Check sheet for the modelled part. Datum: model origin and axes. Units: mm. Face numbers are marked on the shaded views. A direction names the side the tool comes from. Round coordinates to 2 decimals unless told otherwise and drop trailing zeros. Write each loop counter-clockwise with the first axis right and the second up, starting at its lowest first coordinate (ties: lowest second). Pieces come first, ordered by that corner, then holes. Notation, with made-up numbers: (-23.5, 32) - (-13.5, 32) arc R11 ccw to (-13.5, 43) - close; hole circle Ø11 at (65.25, 20). An arc over 180 degrees is marked (long way). Use one line per item in the form item = value. Start each with the question number.
1) Section check B-B (y = -16). Record the boundary of the cut face in (x, z), then the cut area to 3 significant figures.
2) Section check C-C (x = 27). Record the boundary of the cut face in (y, z), then the cut area to 3 significant figures.
3) Section check D-D (y = 5). Record the boundary of the cut face in (x, z) (3 decimals), then the cut area to 3 significant figures.
4) Section check A-A (z = -4). Record the boundary of the cut face in (x, y), then the cut area to 3 significant figures.
5) Gauge pin test, flat ends, axial feed: P1, Ø3, axis at x = 17, z = -0.5, coming from the -Y side; P2, Ø1, axis at x = 33, z = -1, coming from the +Y side; P3, Ø11, axis at y = -14.5, z = 2.5, coming from the -X side; P4, Ø8, axis at x = 26, y = -9, coming from the +Z side. Record the tip position at first contact, or that the pin passes through.
6) Set-up check for the marked faces 1, 2, 3, 4 and 5: record each of +Z, -Z, +X, -X, +Y, -Y from which the full face is reachable in a straight line by a thin tool's end or side.
7) Scan lines: probe 1 along X at (y, z) = (3.25, 0); probe 2 along X at (y, z) = (-1, 0); probe 3 along Z at (x, y) = (17.45, 3.5). Record each from-to range of solid material in increasing order.
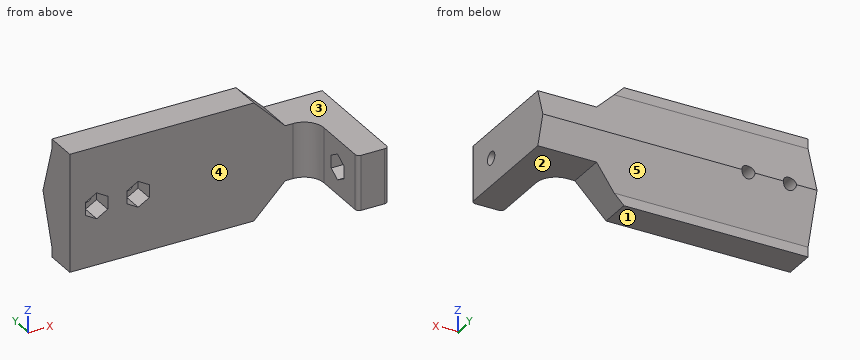
from build123d import *

# Parameters (mm, degrees)
BOSS_EXTRUDE1_DEPTH = 70
SKETCH2_R           = 1.65
CUT_EXTRUDE1_DEPTH  = 5
SKETCH3_R           = 1.65
CUT_EXTRUDE2_DEPTH  = 61
SKETCH4_W           = 8
SKETCH4_H           = 30
BOSS_EXTRUDE2_DEPTH = 20
SKETCH5_R           = 1.65
CUT_EXTRUDE3_DEPTH  = 4
SKETCH6_R           = 1.65
CUT_EXTRUDE4_DEPTH  = 40
FILLET1_R           = 1
FILLET2_R           = 5
SKETCH7_W           = 6
SKETCH7_H           = 8
SKETCH7_W_2         = 1
CUT_EXTRUDE5_DEPTH  = 42
CHAMFER1_SIZE       = 10


with BuildPart() as part:
    # Sketch1 → Boss-Extrude1 (new body)
    with BuildSketch(Plane(origin=(0, 0, 0), x_dir=(0, 0, -1), z_dir=(1, 0, 0))):
        Polygon((0, 8), (12.5, 4), (-12.5, 4), align=None)
        Polygon((12.5, 4), (-12.5, 4), (-15, 4), (-15, -4), (15, -4), (15, 4), align=None)
    extrude(amount=BOSS_EXTRUDE1_DEPTH)

    # Sketch2 → Cut-Extrude1 (cut)
    # profile 1 of 2: a face of its own
    with BuildSketch(Plane.XZ.offset(4)):
        Polygon((6.85, 3.290896534), (4, 1.645448267), (4, -1.645448267), (6.85, -3.290896534), (9.7, -1.645448267), (9.7, 1.645448267), align=None)
        with Locations(Location((6.85, 0, 0), (0, 0, 270))):
            Circle(SKETCH2_R, mode=Mode.SUBTRACT)
    # profile 2 of 2: a face of its own
    with BuildSketch(Plane.XZ.offset(4)):
        Polygon((17.45, -3.290896534), (20.3, -1.645448267), (20.3, 1.645448267), (17.45, 3.290896534), (14.6, 1.645448267), (14.6, -1.645448267), align=None)
        with Locations(Location((17.45, 0, 0), (0, 0, 270))):
            Circle(SKETCH2_R, mode=Mode.SUBTRACT)
    extrude(amount=-CUT_EXTRUDE1_DEPTH, mode=Mode.SUBTRACT)

    # Sketch3 → Cut-Extrude2 (cut)
    with BuildSketch(Plane.XZ.offset(4)):
        with Locations(Location((6.85, 0, 0), (0, 0, 270))):
            Circle(SKETCH3_R)
        with Locations(Location((17.45, 0, 0), (0, 0, 270))):
            Circle(SKETCH3_R)
    extrude(amount=-CUT_EXTRUDE2_DEPTH, mode=Mode.SUBTRACT)

    # Sketch4 → Boss-Extrude2 (add)
    with BuildSketch(Plane.XZ.offset(4)):
        with Locations((66, 0)):
            Rectangle(SKETCH4_W, SKETCH4_H)
    extrude(amount=BOSS_EXTRUDE2_DEPTH)

    # Sketch5 → Cut-Extrude3 (cut)
    with BuildSketch(Plane.ZY.offset(-62)):
        Polygon((3.290896534, -15.15), (1.645448267, -12.3), (-1.645448267, -12.3), (-3.290896534, -15.15), (-1.645448267, -18), (1.645448267, -18), align=None)
        with Locations((0, -15.15)):
            Circle(SKETCH5_R, mode=Mode.SUBTRACT)
    extrude(amount=-CUT_EXTRUDE3_DEPTH, mode=Mode.SUBTRACT)

    # Sketch6 → Cut-Extrude4 (cut)
    with BuildSketch(Plane.ZY.offset(-62)):
        with Locations((0, -15.15)):
            Circle(SKETCH6_R)
    extrude(amount=-CUT_EXTRUDE4_DEPTH, mode=Mode.SUBTRACT)

    # Fillet1
    fillet1_edges = [part.edges().sort_by_distance(p)[0] for p in [
        (70, -24, 0),
        (62, -24, 0),
    ]]
    fillet(fillet1_edges, radius=FILLET1_R)

    # Fillet2
    fillet2_edges = [part.edges().sort_by_distance(p)[0] for p in [
        (62, -4, 0),
    ]]
    fillet(fillet2_edges, radius=FILLET2_R)

    # Sketch7 → Cut-Extrude5 (cut)
    with BuildSketch(Plane.XZ.offset(24)):
        with Locations((66, 11)):
            Rectangle(SKETCH7_W, SKETCH7_H)
        with Locations((69.5, 11)):
            Rectangle(SKETCH7_W_2, SKETCH7_H)
        with Locations((60, 11)):
            Rectangle(SKETCH7_W, SKETCH7_H)
        with Locations((60, -11)):
            Rectangle(SKETCH7_W, SKETCH7_H)
        with Locations((66, -11)):
            Rectangle(SKETCH7_W, SKETCH7_H)
        with Locations((69.5, -11)):
            Rectangle(SKETCH7_W_2, SKETCH7_H)
    extrude(amount=-CUT_EXTRUDE5_DEPTH, mode=Mode.SUBTRACT)

    # Chamfer1
    # the kernel refuses this chamfer: 10 mm, written as the material it takes off along each edge
    with BuildSketch(Plane(origin=(57, -29.71682988, 15), x_dir=(0.027495876610587014, 0, -0.9996219169112968), z_dir=(0, 1, 0))) as chamfer1_piece_1_section:
        Polygon((CHAMFER1_SIZE * 0.999621916911, CHAMFER1_SIZE * 0.0274958766106), (-CHAMFER1_SIZE * 0.0274958766106, CHAMFER1_SIZE * 0.999621916911), (0, 0), align=None)
    chamfer1_piece_1 = extrude(amount=59.433659759, mode=Mode.PRIVATE)
    chamfer1_piece_1 = split(chamfer1_piece_1, bisect_by=Plane(origin=(53.542815877, 0, 7), z_dir=(0, 0, 1)), keep=Keep.TOP, mode=Mode.PRIVATE)
    add(chamfer1_piece_1, mode=Mode.SUBTRACT)
    with BuildSketch(Plane(origin=(57, -29.71682988, -15), x_dir=(-0.9996219169112968, 0, -0.027495876610586317), z_dir=(0, 1, 0))) as chamfer1_piece_2_section:
        Polygon((CHAMFER1_SIZE * 0.999621916911, CHAMFER1_SIZE * 0.0274958766106), (-CHAMFER1_SIZE * 0.0274958766106, CHAMFER1_SIZE * 0.999621916911), (0, 0), align=None)
    chamfer1_piece_2 = extrude(amount=59.433659759, mode=Mode.PRIVATE)
    chamfer1_piece_2 = split(chamfer1_piece_2, bisect_by=Plane(origin=(53.542815877, 0, -7), z_dir=(0, 0, -1)), keep=Keep.TOP, mode=Mode.PRIVATE)
    add(chamfer1_piece_2, mode=Mode.SUBTRACT)


solid = part.part
Results are:
q1.outline = (62, -7) - (70, -7) - (70, -1.41) - (66, -1.41) - (66, -2.8) - (62, -2.8) - close; (62, 2.8) - (66, 2.8) - (66, 1.41) - (70, 1.41) - (70, 7) - (62, 7) - close
q1.area = 78.3 mm²
q2.outline = (-4, -15) - (4, -15) - (4, -12.5) - (8, 0) - (4, 12.5) - (4, 15) - (-4, 15) - close
q2.area = 290 mm²
q3.outline = (0, -9.375) - (52.625, -9.375) - (55, -7) - (70, -7) - (70, 7) - (55, 7) - (52.625, 9.375) - (0, 9.375) - close; hole circle Ø3.3 at (6.85, 0); hole circle Ø3.3 at (17.45, 0)
q3.area = 1,220 mm²
q4.outline = (0, -4) - (57, -4) arc R5 cw to (62, -9) - (62, -23) arc R1 ccw to (63, -24) - (69, -24) arc R1 ccw to (70, -23) - (70, 6.72) - (0, 6.72) - close
q4.area = 915 mm²
q5.P1 = 1
q5.P2 = 7.84
q5.P3 = 62
q5.P4 = through
q6.face_1 = -Z, +X, -X, +Y, -Y
q6.face_2 = -Z, +X, +Y, -Y
q6.face_3 = +Z, +X, +Y, -Y
q6.face_4 = +Z, -Z, -X, -Y
q6.face_5 = -Z, +X, -X, +Y
q7.probe_1 = 0 to 5.2, 8.5 to 15.8, 19.1 to 70
q7.probe_2 = 0 to 4, 9.7 to 14.6, 20.3 to 70
q7.probe_3 = -15 to -1.65, 1.65 to 15
